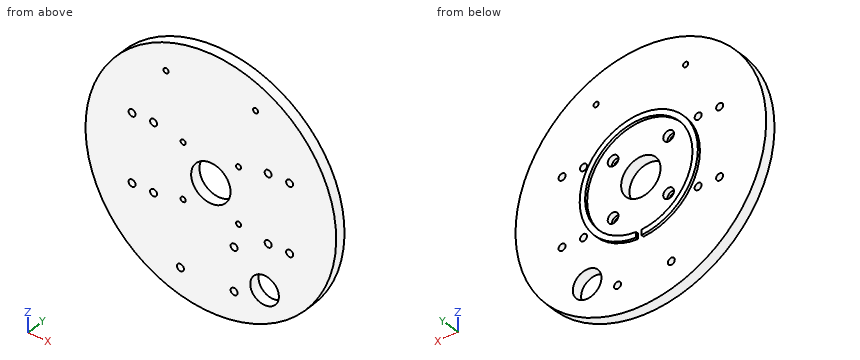
```python
from build123d import *

# Parameters (mm, degrees)
SKETCH1_R           = 70
SKETCH1_R_2         = 11
BOSS_EXTRUDE1_DEPTH = 6
SKETCH2_R           = 1.42
CUT_EXTRUDE2_DEPTH  = 10
SKETCH4_R           = 3
CUT_EXTRUDE3_DEPTH  = 3
SKETCH5_R           = 1.95
CUT_EXTRUDE4_DEPTH  = 10
SKETCH6_R           = 1.95
CUT_EXTRUDE5_DEPTH  = 6
SKETCH7_R           = 1.42
CUT_EXTRUDE6_DEPTH  = 10
SKETCH8_R           = 8
CUT_EXTRUDE7_DEPTH  = 10
SKETCH9_R           = 33
SKETCH9_R_2         = 30
BOSS_EXTRUDE2_DEPTH = 1.5
SKETCH10_W          = 3
SKETCH10_H          = 10.861840942
CUT_EXTRUDE9_DEPTH  = 1.5
SKETCH11_R          = 2.471165228
BOSS_EXTRUDE3_DEPTH = 1


with BuildPart() as part:
    # Sketch1 → Boss-Extrude1 (new body)
    with BuildSketch(Plane(origin=(0, 0, 0), x_dir=(1, 0, 0), z_dir=(0, 1, 0))):
        with Locations(Location((0, 0, 0), (0, 0, 270))):
            Circle(SKETCH1_R)
        with Locations(Location((0, 0, 0), (0, 0, 270))):
            Circle(SKETCH1_R_2, mode=Mode.SUBTRACT)
    extrude(amount=BOSS_EXTRUDE1_DEPTH)

    # Sketch2 → Cut-Extrude2 (cut)
    with BuildSketch(Plane(origin=(0, 6, 0), x_dir=(1, 0, 0), z_dir=(0, 1, 0))):
        with Locations(Location((-15.5, 15.5, 0), (0, 0, 270))):
            Circle(SKETCH2_R)
        with Locations(Location((15.5, 15.5, 0), (0, 0, 270))):
            Circle(SKETCH2_R)
        with Locations(Location((15.5, -15.5, 0), (0, 0, 270))):
            Circle(SKETCH2_R)
        with Locations(Location((-15.5, -15.5, 0), (0, 0, 270))):
            Circle(SKETCH2_R)
    extrude(amount=-CUT_EXTRUDE2_DEPTH, mode=Mode.SUBTRACT)

    # Sketch4 → Cut-Extrude3 (cut)
    with BuildSketch(Plane(origin=(0, 6, 0), x_dir=(1, 0, 0), z_dir=(0, 1, 0))):
        with Locations(Location((-15.5, 15.5, 0), (0, 0, 270))):
            Circle(SKETCH4_R)
        with Locations(Location((15.5, 15.5, 0), (0, 0, 270))):
            Circle(SKETCH4_R)
        with Locations(Location((15.5, -15.5, 0), (0, 0, 270))):
            Circle(SKETCH4_R)
        with Locations(Location((-15.5, -15.5, 0), (0, 0, 270))):
            Circle(SKETCH4_R)
    extrude(amount=-CUT_EXTRUDE3_DEPTH, mode=Mode.SUBTRACT)

    # Sketch5 → Cut-Extrude4 (cut)
    with BuildSketch(Plane(origin=(0, 6, 0), x_dir=(1, 0, 0), z_dir=(0, 1, 0))):
        with Locations(Location((-32, 19, 0), (0, 0, 270))):
            Circle(SKETCH5_R)
        with Locations(Location((-44, 19, 0), (0, 0, 270))):
            Circle(SKETCH5_R)
        with Locations(Location((-44, -19, 0), (0, 0, 270))):
            Circle(SKETCH5_R)
        with Locations(Location((-32, -19, 0), (0, 0, 270))):
            Circle(SKETCH5_R)
        with Locations(Location((32, -19, 0), (0, 0, 270))):
            Circle(SKETCH5_R)
        with Locations(Location((44, -19, 0), (0, 0, 270))):
            Circle(SKETCH5_R)
        with Locations(Location((44, 19, 0), (0, 0, 270))):
            Circle(SKETCH5_R)
        with Locations(Location((32, 19, 0), (0, 0, 270))):
            Circle(SKETCH5_R)
    extrude(amount=-CUT_EXTRUDE4_DEPTH, mode=Mode.SUBTRACT)

    # Sketch6 → Cut-Extrude5 (cut)
    with BuildSketch(Plane(origin=(0, 6, 0), x_dir=(1, 0, 0), z_dir=(0, 1, 0))):
        with Locations(Location((13, 29, 0), (0, 0, 270))):
            Circle(SKETCH6_R)
        with Locations(Location((13, 53, 0), (0, 0, 270))):
            Circle(SKETCH6_R)
        with Locations(Location((-17, 52.999810288, 0), (0, 0, 270))):
            Circle(SKETCH6_R)
    extrude(amount=-CUT_EXTRUDE5_DEPTH, mode=Mode.SUBTRACT)

    # Sketch7 → Cut-Extrude6 (cut)
    with BuildSketch(Plane(origin=(0, 6, 0), x_dir=(1, 0, 0), z_dir=(0, 1, 0))):
        with Locations(Location((-25, -50, 0), (0, 0, 270))):
            Circle(SKETCH7_R)
        with Locations(Location((25, -50, 0), (0, 0, 270))):
            Circle(SKETCH7_R)
    extrude(amount=-CUT_EXTRUDE6_DEPTH, mode=Mode.SUBTRACT)

    # Sketch8 → Cut-Extrude7 (cut)
    with BuildSketch(Plane(origin=(0, 6, 0), x_dir=(1, 0, 0), z_dir=(0, 1, 0))):
        with Locations(Location((30, 45, 0), (0, 0, 270))):
            Circle(SKETCH8_R)
    extrude(amount=-CUT_EXTRUDE7_DEPTH, mode=Mode.SUBTRACT)

    # Sketch9 → Boss-Extrude2 (add)
    with BuildSketch(Plane(origin=(0, 6, 0), x_dir=(1, 0, 0), z_dir=(0, 1, 0))):
        with Locations(Location((0, 0, 0), (0, 0, 68.546799355))):
            Circle(SKETCH9_R)
        with Locations(Location((0, 0, 0), (0, 0, 67.330047366))):
            Circle(SKETCH9_R_2, mode=Mode.SUBTRACT)
    extrude(amount=BOSS_EXTRUDE2_DEPTH)

    # Sketch10 → Cut-Extrude9 (cut)
    with BuildSketch(Plane(origin=(0, 7.5, 0), x_dir=(1, 0, 0), z_dir=(0, 1, 0))):
        with Locations((0, 31.635111745)):
            Rectangle(SKETCH10_W, SKETCH10_H)
    extrude(amount=-CUT_EXTRUDE9_DEPTH, mode=Mode.SUBTRACT)

    # Sketch11 → Boss-Extrude3 (add)
    with BuildSketch(Plane(origin=(0, 6, 0), x_dir=(1, 0, 0), z_dir=(0, 1, 0))):
        with Locations((13, 29)):
            Circle(SKETCH11_R)
    extrude(amount=-BOSS_EXTRUDE3_DEPTH)


solid = part.part
```
The listing builds one solid part. Answer for the finished solid, in the listing's coordinates (mm). Coordinates: 2 decimals unless noted, no trailing zeros. Write each loop counter-clockwise with the first axis right and the second up, starting at its lowest first coordinate (ties: lowest second). Pieces come first, ordered by that corner, then holes. Notation, with made-up numbers: (77, 70) -> (82, 70) arc R24 cw to (82, 109) -> close; hole circle Ø2 at (-34, 48.25). An arc over 180 degrees is marked (long way). Write each question's results on one line, items separated by ' | '. Start each with the question number.
1) Straight lines are drawn through the part: probe 1 along X at (y, z) = (0.5, -20); probe 2 along X at (y, z) = (1.5, -15.5); probe 3 along Z at (x, y) = (15, 3.25). For each, find the intervals that lie inside material, in ascending order.
2) A cutting plane is placed at A-A (z = 0). Determine the outline of the cut face in (x, y).
3) Flat-ended cylindrical pins translate along their axes: pin 1 Ø2.5 at (x, z) = (-32, -19) entering from -Y; pin 2 Ø1 at (x, y) = (9.5, 4.5) entering from -Z; pin 3 Ø3.5 at (x, z) = (25, 50) entering from +Y; pin 4 Ø2 at (x, y) = (-13.5, 3) entering from +Z. Find the tip coordinate at first contact, or state that the pin passes through.
4) A cutting plane is placed at D-D (z = 35.5). Determine the outline of the cut face in (x, y), then the cut area to 3 significant figures.
5) A cutting plane is placed at C-C (z = -43.5). Determine the outline of the cut face in (x, y).
6) A cutting plane is placed at B-B (x = 44). Determine the outline of the cut face in (y, z), then the cut area to 3 significant figures.
Values follow:
1) probe 1: -67.08 to -45.67, -42.33 to -33.67, -30.33 to 30.33, 33.67 to 42.33, 45.67 to 67.08 | probe 2: -68.26 to -16.92, -14.08 to 14.08, 16.92 to 68.26 | probe 3: -68.37 to -18.46, -12.54 to 12.54, 18.46 to 68.37
2) outline: (-70, 0) -> (-11, 0) -> (-11, 6) -> (-30, 6) -> (-30, 7.5) -> (-33, 7.5) -> (-33, 6) -> (-70, 6) -> close; (11, 0) -> (70, 0) -> (70, 6) -> (33, 6) -> (33, 7.5) -> (30, 7.5) -> (30, 6) -> (11, 6) -> close
3) pin 1: through | pin 2: z = -69.42 | pin 3: y = 6 | pin 4: z = 68.87
4) outline: (-60.33, 0) -> (60.33, 0) -> (60.33, 6) -> (-60.33, 6) -> close | area: 724 mm²
5) outline: (-54.84, 0) -> (22.14, 0) -> (22.14, 6) -> (-54.84, 6) -> close; (37.86, 0) -> (54.84, 0) -> (54.84, 6) -> (37.86, 6) -> close
6) outline: (0, -54.44) -> (6, -54.44) -> (6, -20.95) -> (0, -20.95) -> close; (0, -17.05) -> (6, -17.05) -> (6, 17.05) -> (0, 17.05) -> close; (0, 20.95) -> (6, 20.95) -> (6, 54.44) -> (0, 54.44) -> close | area: 607 mm²
